Autodesk Inventor part; units mm, degrees
ref_plane "YZ Plane" through (0, 0, 0) normal (1, 0, 0) x (0, 1, 0)
ref_plane "XZ Plane" through (0, 0, 0) normal (0, 1, 0) x (-1, 0, 0)
ref_plane "XY Plane" through (0, 0, 0) normal (0, 0, 1) x (1, 0, 0)
sketch "Sketch1" plane through (0, 0, 0) normal (0, 0, 1) x (1, 0, 0)
  line L0 (35, 25) -> (-35, 25)
  line L1 (-35, 25) -> (-35, -25)
  line L2 (-35, -25) -> (35, -25)
  line L3 (35, -25) -> (35, 25)
  line L4 (35, 25) -> (-35, -25) construction
  line L5 (-35, 25) -> (35, -25) construction
  point P0 (0, 0)
  dimension "d0" = 70
  dimension "d1" = 50
extrude "Extrusion1" add sketch "Sketch1" along normal blind 41
sketch "Sketch2" plane through (-35, -25, 0) normal (-1, 0, 0) x (0, 0, 1)
  line L0 (0, 50) -> (23, 50)
  line L1 (0, 50) -> (41, 50)
  line L2 (23, 50) -> (23, 10)
  line L3 (23, 10) -> (3, 10)
  line L4 (3, 10) -> (3, 12.5)
  line L5 (3, 12.5) -> (0, 12.5)
  line L6 (0, 0) -> (41, 0)
  line L7 (0, 50) -> (0, 12.5)
  point P0 (0, 25)
  dimension "d4" = 23
  dimension "d5" = 40
  dimension "d6" = 20
  dimension "d7" = 12.5
extrude "Extrusion2" cut sketch "Sketch2" against normal through all
sketch "Sketch3" plane through (0, 0, 41) normal (0, 0, 1) x (1, 0, 0)
  line L0 (-15, -7) -> (15, -7)
  line L1 (15, -7) -> (15, -25)
  line L2 (15, -25) -> (-15, -25)
  line L3 (-15, -25) -> (-15, -7)
  line L4 (-35, -25) -> (35, -25)
  point P0 (0, 0)
  dimension "d10" = 30
  dimension "d11" = 18
  dimension "d12" = 15
  dimension "d13" = 0
extrude "Extrusion3" cut sketch "Sketch3" against normal through all
sketch "Sketch4" plane through (0, 0, 41) normal (0, 0, 1) x (1, 0, 0)
  line L0 (35, 25) -> (-35, 25)
  point P0 (0, 0)
  point P1 (-22.5, 0)
  point P2 (22.5, 0)
  dimension "d16" = 25
  dimension "d17" = 22.5
  dimension "d18" = 45
  dimension "d19" = 25
hole "Hole1" at (-22.5, 0, 41) at (22.5, 0, 41) direction (0, 0, -1) diameter 8.4 end through all counterbore diameter 15 counterbore depth 8
sketch "Sketch5" plane through (-35, -25, 41) normal (-1, 0, 0) x (0, 0, 1)
  line L0 (0, 50) -> (0, 0)
  line L1 (-41, 0) -> (0, 0)
  point P0 (-41, 25)
  point P1 (-10, 10)
  dimension "d27" = 10
  dimension "d28" = 10
hole "Hole2" at (-35, -15, 31) direction (1, 0, 0) diameter 8 end through all
chamfer "Chamfer1" distance 2 angle 45 7 edges at (-35, 0, 41) (-25, -25, 41) (0, 25, 41) (35, 0, 41) (25, -25, 41) (-35, -25, 20.5) (35, -25, 20.5)
properties part number "Lager" material "Iron, Cast"
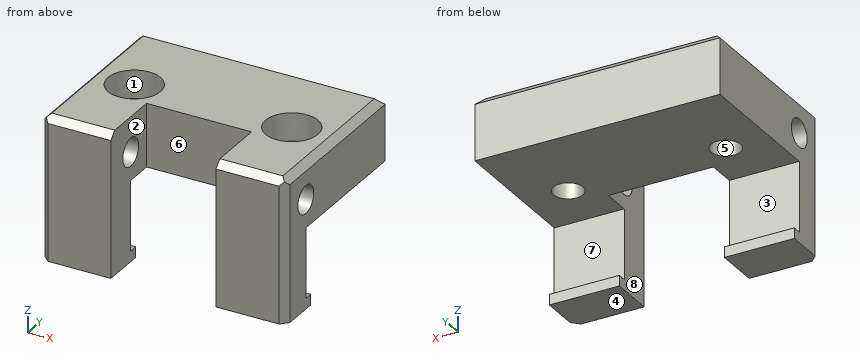
Can you work these out from the model? Positions are in its coordinate system, mm. Face numbers are marked on the shaded views. A direction names the side the tool comes from. Give positions to 0.01 mm unless a question says otherwise; leave off trailing zeros. Order: outer loops, then holes, each group sorted by start corner. A loop starts at its lowest first (then second) coordinate and runs counter-clockwise, first axis right, second up. Notation, with made-up numbers: M -1,53.25 L 28,53.25 A17 cw 28,63.25 Z; hole C 75,-24.5 d10. An arc over 180 degrees is marked long. Use a Markdown table: item, result. Add a question column.
Item 1: Suppose I cut it at B-B (y = 0). List the corners of the cut face in (x, z) for me, then the cut area to 3 significant figures.
Item 2: We'd pull the mould along Y, two halves only. Please class the marked faces 5, 6, 7 and 8: +Y half, -Y half, draft (parallel to the pull), parting line (faces both ways), or undercut.
Item 3: Suppose I cut it at D-D (z = 15). List the corners of the cut face in (x, y) for me, then the cut area to 3 significant figures.
Item 4: For the marked faces 1, 2, 3 and 4, which set-ups out of +Z, -Z, +X, -X, +Y, -Y let a thin tool reach every point of the face, with its end or its side?
Item 5: Suppose I cut it at A-A (z = 31). List the corners of the cut face in (x, y) for me, then the cut area to 3 significant figures.
Item 6: Suppose I cut it at C-C (x = 22.5). List the corners of the cut face in (y, z) for me, then the cut area to 3 significant figures.
Item 7: If I drill on L1, parallel to X at y = 0, z = 30.5; L2, parallel to Y at x = 22.5, z = 25.75; L3, parallel to Y at x = 24.75, z = 31, over which ranges is the centre line in solid material (lowest first)? Write a range as [from, to].
Item 8: Will these pins go through, and if not, where does the flat tip stop? pin 1 (1.5 mm diameter, centred on y = 5, z = 22, fed in from +X) (1 decimal); pin 2 (22 mm diameter, centred on x = -29, z = 11.5, fed in from +Y); pin 3 (1 mm diameter, centred on x = 24, y = -15, fed in from -Z); pin 4 (1.5 mm diameter, centred on x = -9, y = 12, fed in from -Z).
Answer sheet:
| question | item | result |
|---|---|---|
| 1 | outline | M -35,23 L -26.7,23 L -26.7,33 L -30,33 L -30,41 L -33,41 L -35,39 Z; M -18.3,23 L 18.3,23 L 18.3,33 L 15,33 L 15,41 L -15,41 L -15,33 L -18.3,33 Z; M 26.7,23 L 35,23 L 35,39 L 33,41 L 30,41 L 30,33 L 26.7,33 Z |
| 1 | area | 848 mm² |
| 2 | face 5 | undercut |
| 2 | face 6 | -Y half |
| 2 | face 7 | +Y half |
| 2 | face 8 | draft |
| 3 | outline | M -35,-23 L -33,-25 L -15,-25 L -15,-15 L -35,-15 Z; M 15,-25 L 33,-25 L 35,-23 L 35,-15 L 15,-15 Z |
| 3 | area | 396 mm² |
| 4 | face 1 | +Z |
| 4 | face 2 | +Z, -Z, -Y |
| 4 | face 3 | +X, -X, +Y |
| 4 | face 4 | -Z, +X, -X, +Y, -Y |
| 5 | outline | M -35,-23 L -33,-25 L -15,-25 L -15,-19 L -35,-19 Z; M -35,-11 L -15,-11 L -15,-7 L 15,-7 L 15,-11 L 35,-11 L 35,25 L -35,25 Z; M 15,-25 L 33,-25 L 35,-23 L 35,-19 L 15,-19 Z; hole C -22.5,0 d8.4; hole C 22.5,0 d8.4 |
| 5 | area | 2,530 mm² |
| 6 | outline | M -25,0 L -12.5,0 L -12.5,3 L -15,3 L -15,23 L -4.2,23 L -4.2,33 L -7.5,33 L -7.5,41 L -23,41 L -25,39 Z; M 4.2,23 L 25,23 L 25,39 L 23,41 L 7.5,41 L 7.5,33 L 4.2,33 Z; hole C -15,31 d8 |
| 6 | area | 879 mm² |
| 7 | L1 | x = [-35, -26.7], [-18.3, 18.3], [26.7, 35] |
| 7 | L2 | y = [-25, -4.2], [4.2, 25] |
| 7 | L3 | y = [-25, -19], [-11, -3.55], [3.55, 25] |
| 8 | pin 1 | passes through |
| 8 | pin 2 | stops at y = -12.5 |
| 8 | pin 3 | stops at z = 0 |
| 8 | pin 4 | stops at z = 23 |
